Here's how the part is built. I have some questions about the finished solid (model axes, mm). Face numbers are marked on the shaded views. A direction names the side the tool comes from. Coordinates: 2 decimals unless noted, no trailing zeros. Write each loop counter-clockwise with the first axis right and the second up, starting at its lowest first coordinate (ties: lowest second). Pieces come first, ordered by that corner, then holes. Notation, with made-up numbers: (81, 69) -> (125, 69) arc R24 ccw to (125, 86) -> close; hole circle Ø7 at (74.5, 71). An arc over 180 degrees is marked (long way). Use CSV: the item, a comma, the result in double quotes. Start each with the question number.
```python
from build123d import *

# Parameters (mm, degrees)
SKETCH2_W           = 25
SKETCH2_H           = 42
BOSS_EXTRUDE1_DEPTH = 4
SKETCH5_W           = 56
SKETCH5_H           = 15
BOSS_EXTRUDE2_DEPTH = 25
BOSS_EXTRUDE3_DEPTH = 3
SKETCH7_W           = 1.5
SKETCH7_H           = 10.5
CUT_EXTRUDE1_DEPTH  = 69.353858706
SKETCH9_R           = 2
CUT_EXTRUDE2_DEPTH  = 6
CHAMFER1_SIZE       = 10.5
SKETCH10_R          = 1
CUT_EXTRUDE3_DEPTH  = 66.117202028
SKETCH11_W          = 20.5
SKETCH11_H          = 19.25
CUT_EXTRUDE4_DEPTH  = 66.117202028
CHAMFER3_SIZE       = 1.5
SKETCH12_R          = 3
CUT_EXTRUDE5_DEPTH  = 66.117202028
CHAMFER4_SIZE       = 1
SKETCH13_R          = 2
CUT_EXTRUDE6_DEPTH  = 1.5
CUT_EXTRUDE7_DEPTH  = 73.221880341
FILLET1_R           = 2
SKETCH16_W          = 12
SKETCH16_H          = 45
CUT_EXTRUDE8_DEPTH  = 4.5
CHAMFER5_SIZE       = 4.5


with BuildPart() as part:
    # Sketch2 → Boss-Extrude1 (new body)
    with BuildSketch(Plane.XY):
        Rectangle(SKETCH2_W, SKETCH2_H)
    extrude(amount=BOSS_EXTRUDE1_DEPTH)

    # Sketch5 → Boss-Extrude2 (add, through all)
    with BuildSketch(Plane(origin=(12.5, 0, 0), x_dir=(0, 0, -1), z_dir=(1, 0, 0))):
        with Locations((-28, -28.5)):
            Rectangle(SKETCH5_W, SKETCH5_H)
    extrude(amount=-BOSS_EXTRUDE2_DEPTH)

    # Sketch6 → Boss-Extrude3 (add)
    with BuildSketch(Plane(origin=(12.5, 0, 0), x_dir=(0, 0, -1), z_dir=(1, 0, 0))):
        Polygon((-4, 21), (0, 21), (0, -36), (-56, -36), (-56, -21), (-51, -21), align=None)
    boss_extrude3 = extrude(amount=BOSS_EXTRUDE3_DEPTH)

    # Sketch7 → Cut-Extrude1 (cut, through all)
    with BuildSketch(Plane.XY.offset(56)):
        with Locations((14.75, -30.75)):
            Rectangle(SKETCH7_W, SKETCH7_H)
    cut_extrude1 = extrude(amount=-CUT_EXTRUDE1_DEPTH, mode=Mode.SUBTRACT)

    # Sketch9 → Cut-Extrude2 (cut)
    with BuildSketch(Plane(origin=(14, 0, 0), x_dir=(0, 0, -1), z_dir=(1, 0, 0))):
        with Locations((-51, -31)):
            Circle(SKETCH9_R)
        with Locations((-16, -31)):
            Circle(SKETCH9_R)
    cut_extrude2 = extrude(amount=-CUT_EXTRUDE2_DEPTH, mode=Mode.SUBTRACT)

    # Mirror1: Boss-Extrude3, Cut-Extrude1, Cut-Extrude2 across plane
    add(boss_extrude3.mirror(Plane(origin=(0, 0, 0), x_dir=(0, 0, 1), z_dir=(1, 0, 0))))
    add(cut_extrude1.mirror(Plane(origin=(0, 0, 0), x_dir=(0, 0, 1), z_dir=(1, 0, 0))), mode=Mode.SUBTRACT)
    add(cut_extrude2.mirror(Plane(origin=(0, 0, 0), x_dir=(0, 0, 1), z_dir=(1, 0, 0))), mode=Mode.SUBTRACT)

    # Chamfer1
    chamfer1_edges = [part.edges().sort_by_distance(p)[0] for p in [
        (0, -36, 0),
    ]]
    chamfer(chamfer1_edges, length=CHAMFER1_SIZE)

    # Sketch10 → Cut-Extrude3 (cut, through all)
    with BuildSketch(Plane.XY.offset(4)):
        with Locations((-10.25, 5.7)):
            Circle(SKETCH10_R)
        with Locations((10.25, 5.7)):
            Circle(SKETCH10_R)
        with Locations((10.25, -18.75)):
            Circle(SKETCH10_R)
        with Locations((-10.25, -18.75)):
            Circle(SKETCH10_R)
    extrude(amount=-CUT_EXTRUDE3_DEPTH, mode=Mode.SUBTRACT)

    # Sketch11 → Cut-Extrude4 (cut, through all)
    with BuildSketch(Plane.XY.offset(4)):
        with Locations((0, -6.375)):
            Rectangle(SKETCH11_W, SKETCH11_H)
    extrude(amount=-CUT_EXTRUDE4_DEPTH, mode=Mode.SUBTRACT)

    # Chamfer3
    chamfer3_edges = [part.edges().sort_by_distance(p)[0] for p in [
        (10.25, 3.25, 2),
        (10.25, -16, 2),
        (-10.25, -16, 2),
        (-10.25, 3.25, 2),
    ]]
    chamfer(chamfer3_edges, length=CHAMFER3_SIZE)

    # Sketch12 → Cut-Extrude5 (cut, through all)
    with BuildSketch(Plane.XY.offset(4)):
        with Locations((0, 14)):
            Circle(SKETCH12_R)
    extrude(amount=-CUT_EXTRUDE5_DEPTH, mode=Mode.SUBTRACT)

    # Chamfer4
    chamfer4_edges = [part.edges().sort_by_distance(p)[0] for p in [
        (-3, 14, 0),
        (-3, 14, 4),
    ]]
    chamfer(chamfer4_edges, length=CHAMFER4_SIZE)

    # Sketch13 → Cut-Extrude6 (cut)
    with BuildSketch(Plane(origin=(0, 0, 0), x_dir=(-1, 0, 0), z_dir=(0, 0, -1))):
        with Locations((-10.25, 5.7)):
            Circle(SKETCH13_R)
        with Locations((10.25, 5.7)):
            Circle(SKETCH13_R)
        with Locations((10.25, -18.75)):
            Circle(SKETCH13_R)
        with Locations((-10.25, -18.75)):
            Circle(SKETCH13_R)
    extrude(amount=-CUT_EXTRUDE6_DEPTH, mode=Mode.SUBTRACT)

    # Sketch14 → Cut-Extrude7 (cut, through all)
    with BuildSketch(Plane(origin=(-12.5, 0, 0), x_dir=(0, 0, -1), z_dir=(1, 0, 0))):
        Polygon((-35.28118028, -15), (-10, -15), (-10, 7.591693017), align=None)
    cut_extrude7 = extrude(amount=-CUT_EXTRUDE7_DEPTH, mode=Mode.SUBTRACT)

    # Mirror2: Cut-Extrude7 across plane
    add(cut_extrude7.mirror(Plane(origin=(0, 0, 0), x_dir=(0, 0, 1), z_dir=(1, 0, 0))), mode=Mode.SUBTRACT)

    # Fillet1
    fillet1_edges = [part.edges().sort_by_distance(p)[0] for p in [
        (-14, -15, 35.28118028),
        (-14, 7.591693017, 10),
        (-14, -15, 10),
        (14, 7.591693017, 10),
        (14, -15, 35.28118028),
        (14, -15, 10),
    ]]
    fillet(fillet1_edges, radius=FILLET1_R)

    # Sketch16 → Cut-Extrude8 (cut)
    with BuildSketch(Plane(origin=(0, -21, 0), x_dir=(1, 0, 0), z_dir=(0, 1, 0))):
        with Locations((0, -22.5)):
            Rectangle(SKETCH16_W, SKETCH16_H)
    extrude(amount=-CUT_EXTRUDE8_DEPTH, mode=Mode.SUBTRACT)

    # Chamfer5
    chamfer5_edges = [part.edges().sort_by_distance(p)[0] for p in [
        (0, -25.5, 45),
    ]]
    chamfer(chamfer5_edges, length=CHAMFER5_SIZE - 0.0001)  # a hair under: the kernel refuses the full size


solid = part.part
```
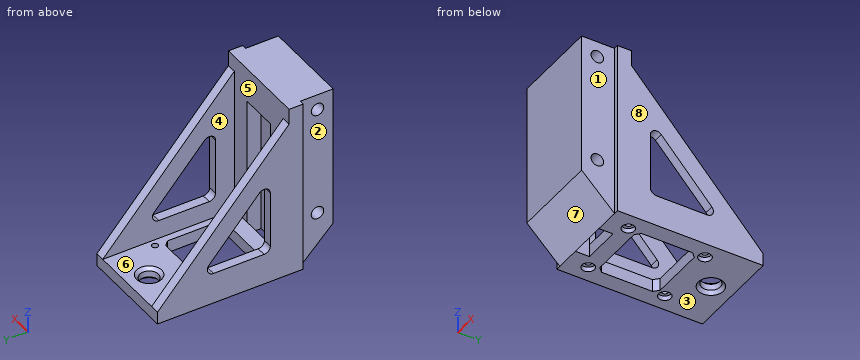
Item 1: If I drill on line 1 along Y through (x, z) = (10.1, 16); line 2 along X through (y, z) = (0.5, 24.5); line 3 along X through (y, z) = (-18, 2), over which ranges is the centre line in solid material (lowest first)?
Item 2: I want a section at A-A on y = 14. Please give me the cut outline in (x, z), then the cut area to 3 significant figures.
Item 3: Thinking about a two-plate mould opening in X: for the marked faces 5, 6, 7 and 8, which applies, +X half, -X half, draft (parallel to the pull), parting line (faces both ways), or undercut?
Item 4: Which directions (+Z, -Z, +X, -X, +Y, -Y) give clear straight access to the entire face, cutting with the end or side of a thin tool? Please do the marked faces 1, 2, 3 and 4.
Item 5: I want a section at B-B on z = 16. Count the separate pieces of the cut face and the enclosed holes in it, then the cut area to 3 significant figures.
Item 6: I want a section at C-C on y = -31. Please give me the cut outline in (x, z).
Item 7: I want a section at D-D on y = -2. Please give me the cut outline in (x, z).
Item 8: I'm going to push flat-ended pins straight in: pin 1 (2.5 mm diameter, centred on x = -10.25, y = -18.75, fed in from +Z); pin 2 (1.2 mm diameter, centred on x = 1, z = 2.5, fed in from -Y); pin 3 (3 mm diameter, centred on y = -31, z = 16, fed in from +X). Where does each tip first touch, or does it pass through?
Geometry says:
1,line 1,"-36 to -33, -29 to -21"
1,line 2,"-15.5 to -12.5, 12.5 to 15.5"
1,line 3,"-15.5 to -10.91, -9.59 to 9.59, 10.91 to 15.5"
2,outline,"(-15.5, 0) -> (-4, 0) -> (-3, 1) -> (-3, 3) -> (-4, 4) -> (-12.5, 4) -> (-12.5, 11.83) -> (-15.5, 11.83) -> close; (3, 1) -> (4, 0) -> (15.5, 0) -> (15.5, 11.83) -> (12.5, 11.83) -> (12.5, 4) -> (4, 4) -> (3, 3) -> close"
2,area,"145 mm2"
3,face 5,"undercut"
3,face 6,"undercut"
3,face 7,"draft"
3,face 8,"+X half"
4,face 1,"+Z, -Z, +X, -Y"
4,face 2,"+Z, -Z, -X, -Y"
4,face 3,"-Z, +X, -X, +Y, -Y"
4,face 4,"+Z, +Y"
5,separate pieces,"3"
5,enclosed holes,"0"
5,area,"416 mm2"
6,outline,"(-14, 5.5) -> (14, 5.5) -> (14, 14) -> (8, 14) -> (8, 18) -> (14, 18) -> (14, 49) -> (8, 49) -> (8, 53) -> (14, 53) -> (14, 56) -> (-14, 56) -> (-14, 53) -> (-8, 53) -> (-8, 49) -> (-14, 49) -> (-14, 18) -> (-8, 18) -> (-8, 14) -> (-14, 14) -> close"
7,outline,"(-15.5, 0) -> (-10.25, 0) -> (-10.25, 4) -> (-12.5, 4) -> (-12.5, 10) -> (-15.5, 10) -> close; (-15.5, 20.73) -> (-12.5, 20.73) -> (-12.5, 29.74) -> (-15.5, 29.74) -> close; (10.25, 0) -> (15.5, 0) -> (15.5, 10) -> (12.5, 10) -> (12.5, 4) -> (10.25, 4) -> close; (12.5, 20.73) -> (15.5, 20.73) -> (15.5, 29.74) -> (12.5, 29.74) -> close"
8,pin 1,"z = 4"
8,pin 2,"y = -28.6"
8,pin 3,"x = 8"
